```python
from build123d import *

# Parameters (mm, degrees)
SKETCH_2_R          = 36.366400699
CUT_EXTRUDE_1_DEPTH = 16
SKETCH_3_R          = 34.490812752
EXTRUDE_1_DEPTH     = 1


with BuildPart() as part:
    # 草图1 → 旋转1 (revolve)
    with BuildSketch(Plane.XY):
        with BuildLine():
            Line((-38.083747267, -28.5), (-32.083747267, -28.5))
            ThreePointArc((-32.083747267, -28.5), (-30.669533704, -29.085786438), (-30.083747267, -30.5))
            Line((-30.083747267, -30.5), (-30.083747267, -44))
            ThreePointArc((-30.083747267, -44), (-29.790854048, -44.707106781), (-29.083747267, -45))
            Line((-29.083747267, -45), (-27.565467955, -45))
            ThreePointArc((-27.565467955, -45), (-26.713721936, -45.190434107), (-26.02417741, -45.72547128))
            Line((-26.02417741, -45.72547128), (-25.083747267, -46.86273564))
            Line((-25.083747267, -46.86273564), (-25.854392539, -47.5))
            Line((-25.854392539, -47.5), (-26.494868211, -46.72547128))
            ThreePointArc((-26.494868211, -46.72547128), (-27.184412737, -46.190434107), (-28.036158755, -46))
            Line((-28.036158755, -46), (-30.083747267, -46))
            ThreePointArc((-30.083747267, -46), (-30.790854048, -45.707106781), (-31.083747267, -45))
            Line((-31.083747267, -45), (-31.083747267, -31.5))
            ThreePointArc((-31.083747267, -31.5), (-31.669533704, -30.085786438), (-33.083747267, -29.5))
            Line((-33.083747267, -29.5), (-37.083747267, -29.5))
            ThreePointArc((-37.083747267, -29.5), (-37.790854048, -29.207106781), (-38.083747267, -28.5))
        make_face()
    revolve(axis=Axis((-28.083747267, 0, 0), (1, 0, 0)))

    # 草图2 → 切除-拉伸1 (cut)
    with BuildSketch(Plane.ZY.offset(31.083747267)):
        Circle(SKETCH_2_R)
    extrude(amount=CUT_EXTRUDE_1_DEPTH, mode=Mode.SUBTRACT)

    # 草图3 → 凸台-拉伸1 (add)
    with BuildSketch(Plane.ZY.offset(31.083747267)):
        Circle(SKETCH_3_R)
    extrude(amount=-EXTRUDE_1_DEPTH)


solid = part.part
```
CAD build for the part. Positions are in the model's coordinates, mm. Give positions to 0.01 mm unless a question says otherwise; leave off trailing zeros. Order: outer loops, then holes, each group sorted by start corner. A loop starts at its lowest first (then second) coordinate and runs counter-clockwise, first axis right, second up.
(1) Flat gauge pins, fed straight in: pin 1 (8 mm diameter, centred on y = -11, z = 22.5, fed in from +X); pin 2 (1 mm diameter, centred on x = -29.5, y = -5, fed in from -Z). Where does each tip first touch, or does it go through?
(2) Drill centre lines: L1, parallel to Y at x = -28, z = 0; L2, parallel to X at y = -18.5, z = 20.5. Where is each one in solid material? Low to high.
(3) Mould opens along Y. For faces 1 (the cylindrical face through (-28.314, -20.765, 39.923)), 2 (the flat face through (-30.084, -1, -1)), 3 (the flat face through (-31.084, 1, -1)), 4 (the cylindrical face through (-29.07, 5.99, -45.61)) say: released by +Y, released by -Y, zero draft, split by the parting line, or undercut.
(4) Saw through at A-A, the plane z = 0. Give the cut face in (x, y).
Results found:
1. pin 1: stops at x = -30.08
1. pin 2: stops at z = -45.78
2. L1: y = -46 to -45, 45 to 46
2. L2: x = -31.08 to -30.08
3. face 1: undercut
3. face 2: undercut
3. face 3: zero draft
3. face 4: split by the parting line
4. outline: (-31.08, -45) arc R1 ccw to (-30.08, -46) - (-28.04, -46) arc R2 cw to (-26.49, -46.73) - (-25.85, -47.5) - (-25.08, -46.86) - (-26.02, -45.73) arc R2 ccw to (-27.57, -45) - (-29.08, -45) arc R1 cw to (-30.08, -44) - (-30.08, 44) arc R1 cw to (-29.08, 45) - (-27.57, 45) arc R2 ccw to (-26.02, 45.73) - (-25.08, 46.86) - (-25.85, 47.5) - (-26.49, 46.73) arc R2 cw to (-28.04, 46) - (-30.08, 46) arc R1 ccw to (-31.08, 45) - close
